Could you check a few things on this model? Use its own coordinates, in mm. A direction names the side the tool comes from. Coordinates: 2 decimals unless noted, no trailing zeros. Order: outer loops, then holes, each group sorted by start corner. A loop starts at its lowest first (then second) coordinate and runs counter-clockwise, first axis right, second up. Notation, with made-up numbers: (5, -23.75) - (31, -23.75) arc R18 ccw to (31, 4.25) - close; hole circle Ø1 at (65.5, 53.25). An arc over 180 degrees is marked (long way). Answer as a JSON object with one key per item and string values. Group by question number.
(1) We'd pull the mould along Y, two halves only. Please class faces 1 (the flat face through (394, 0, 251)), 2 (the flat face through (394, -42, 1040)), 3 (the flat face through (394, -177, 2000)): pulls with the +Y half, pulls with the -Y half, needs draft (parallel to the pull), parting line crosses it, or undercut.
(2) Will these pins go through, and if not, where does the flat tip stop? P1, Ø1.5, axis at x = 508.5, z = 1245.5, coming from the -Y side; P2, Ø9.5, axis at x = 518, z = 1723, coming from the -Y side; P3, Ø4.5, axis at x = 214.5, z = 849, coming from the -Y side.
(3) Imagine slicing it at B-B, the plane z = 1102. Write out the boundary of the cut face in (x, y), and give its area (3 significant figures).
(4) Imagine slicing it at A-A, the plane y = -397. Write out the boundary of the cut face in (x, z).
(5) Please list where these lines run through material, in increasing order: probe 1 along Y at (x, z) = (148, 1897); probe 2 along Y at (x, z) = (254, 1724.5); probe 3 along Y at (x, z) = (695.5, 951).
(6) Which directions (+Z, -Z, +X, -X, +Y, -Y) give clear straight access to the entire face, cutting with the end or side of a thin tool? Please do faces 4 (the flat face through (394, -42, 1565)), 5 (the flat face through (394, 0, 1651)).
from build123d import *

# Parameters (mm, degrees)
BOSS_EXTRUDE1_DEPTH = 800
CUT_EXTRUDE1_REACH  = 2376.868
LPATTERN1_COUNT     = 11
LPATTERN1_PITCH     = 175


with BuildPart() as part:
    # Sketch4 → Boss-Extrude1 (new body)
    with BuildSketch(Plane(origin=(0, 0, 0), x_dir=(0, 0, -1), z_dir=(1, 0, 0))):
        Polygon((0, 0), (-2000, 0), (-2000, -360), (-300, -1000), (0, -1000), align=None)
    extrude(amount=BOSS_EXTRUDE1_DEPTH)

    # Sketch6 → Cut-Extrude1 (cut, up to next)
    with BuildSketch(Plane(origin=(0, 0, 0), x_dir=(0, 0, -1), z_dir=(1, 0, 0)), mode=Mode.PRIVATE) as cut_extrude1_sk1:
        Polygon((-154, 0), (-176, 0), (-176, -25.3), (-184.85, -25.3), (-184.85, -42), (-145.15, -42), (-145.15, -25.3), (-154, -25.3), align=None)
    cut_extrude1_tool1 = extrude(cut_extrude1_sk1.sketch, amount=CUT_EXTRUDE1_REACH, mode=Mode.PRIVATE) & part.part
    cut_extrude1 = cut_extrude1_tool1.solids().sort_by_distance((0, -24.065959, 165))[0]
    add(cut_extrude1, mode=Mode.SUBTRACT)

    # LPattern1: Cut-Extrude1 ×11
    with Locations(*[(0, 0, i * LPATTERN1_PITCH) for i in range(1, LPATTERN1_COUNT)]):
        add(cut_extrude1, mode=Mode.SUBTRACT)


solid = part.part
Result set:
{
 "1": {"face 1": "pulls with the +Y half", "face 2": "undercut", "face 3": "needs draft"},
 "2": {"P1": "stops at y = -644.33", "P2": "stops at y = -466.07", "P3": "stops at y = -794.16"},
 "3": {"outline": "(0, -698.07) - (800, -698.07) - (800, 0) - (0, 0) - close", "area": "558,000 mm^2"},
 "4": {"outline": "(0, 0) - (800, 0) - (800, 1901.72) - (0, 1901.72) - close"},
 "5": {"probe 1": "y = -398.78 to -42, -25.3 to 0", "probe 2": "y = -463.72 to -42, -25.3 to 0", "probe 3": "y = -754.92 to 0"},
 "6": {"face 4": "+X, -X", "face 5": "+Z, -Z, +X, -X, +Y"}
}
